Autodesk Inventor part; units mm, degrees
ref_plane "YZ Plane" through (0, 0, 0) normal (1, 0, 0) x (0, 1, 0)
ref_plane "XZ Plane" through (0, 0, 0) normal (0, 1, 0) x (-1, 0, 0)
ref_plane "XY Plane" through (0, 0, 0) normal (0, 0, 1) x (1, 0, 0)
sketch "Sketch1" plane through (0, 0, 0) normal (0, 0, 1) x (1, 0, 0)
  line L0 (-115, 162.5) -> (115, 162.5)
  line L1 (115, 162.5) -> (115, -162.5)
  line L2 (115, -162.5) -> (-115, -162.5)
  line L3 (-115, -162.5) -> (-115, 162.5)
  point P0 (0, 0)
  point P1 (0, 162.5)
  point P2 (-115, 0)
  dimension "d0" = 230
  dimension "d1" = 325
extrude "Extrusion1" add sketch "Sketch1" along normal blind 8
sketch "Sketch2" plane through (0, 0, 8) normal (0, 0, 1) x (1, 0, 0)
  line L0 (-110, -157.5) -> (110, -157.5) construction
  line L1 (110, -157.5) -> (110, 157.5) construction
  line L2 (110, 157.5) -> (-110, 157.5) construction
  line L3 (-110, 157.5) -> (-110, -157.5) construction
  line L4 (-115, 162.5) -> (-115, -162.5) construction
  line L5 (115, 162.5) -> (-115, 162.5) construction
  point P0 (0, 0)
  point P1 (-110, 0)
  point P2 (-115, 0)
  point P3 (-115, 0)
  point P4 (0, 157.5)
  point P5 (0, 162.5)
  dimension "d4" = 5
  dimension "d5" = 5
hole "Hole1" at (-110, -157.5, 8) at (-110, 157.5, 8) at (110, 157.5, 8) at (110, -157.5, 8) direction (0, 0, -1) diameter 3.5 end through all
sketch "Sketch3" plane through (0, 0, 8) normal (0, 0, 1) x (1, 0, 0)
  line L0 (65, -162.5) -> (-65, -162.5)
  line L1 (-65, -162.5) -> (-65, -25)
  line L2 (-65, -25) -> (65, -25)
  line L3 (65, -25) -> (65, -162.5)
  line L4 (-115, -162.5) -> (115, -162.5)
  line L5 (115, -162.5) -> (115, 162.5)
  line L6 (-115, 162.5) -> (-115, -162.5)
  line L7 (65, 25) -> (-65, 25)
  line L8 (-65, 25) -> (-65, 162.5)
  line L9 (-65, 162.5) -> (65, 162.5)
  line L10 (65, 162.5) -> (65, 25)
  line L11 (115, 162.5) -> (-115, 162.5)
  point P0 (0, 0)
  dimension "d13" = 50
  dimension "d14" = 50
  dimension "d15" = 25
  dimension "d16" = 25
extrude "Extrusion2" cut sketch "Sketch3" against normal blind 10 contours L0 L1 L2 L3 | L10 L7 L8 L9
sketch "Sketch4" plane through (0, 0, 8) normal (0, 0, 1) x (1, 0, 0)
  line L0 (-10, -15) -> (10, -15)
  line L1 (10, -15) -> (10, -5)
  line L2 (10, -5) -> (-10, -5)
  line L3 (-10, -5) -> (-10, -15)
  line L4 (-10, 5) -> (10, 5)
  line L5 (10, 5) -> (10, 15)
  line L6 (10, 15) -> (-10, 15)
  line L7 (-10, 15) -> (-10, 5)
  line L8 (-65, -25) -> (65, -25)
  line L9 (65, 25) -> (-65, 25)
  point P0 (0, 0)
  point P1 (0, -5)
  point P2 (0, 5)
  dimension "d19" = 10
  dimension "d20" = 10
  dimension "d21" = 10
  dimension "d22" = 20
extrude "Extrusion3" cut sketch "Sketch4" against normal through all
properties part number "0005-10-014 Suport Bed"
The model under review builds one solid part; all positions refer to its coordinate system, in mm. A direction names the side the tool comes from. Coordinates: 2 decimals unless noted, no trailing zeros. Order: outer loops, then holes, each group sorted by start corner. A loop starts at its lowest first (then second) coordinate and runs counter-clockwise, first axis right, second up. Notation, with made-up numbers: (69.25, 36) -> (107.25, 36) arc R11 ccw to (107.25, 48) -> close; hole circle Ø8 at (53, 63.5). An arc over 180 degrees is marked (long way). Answer in a Markdown table with one row per item.
(1) Consider section C-C (z = 5.75). Write out the cut boundary in (x, y), plus the area to 3 significant figures.
Answers:
| item | result |
|---|---|
| outline | (-115, -162.5) -> (-65, -162.5) -> (-65, -25) -> (65, -25) -> (65, -162.5) -> (115, -162.5) -> (115, 162.5) -> (65, 162.5) -> (65, 25) -> (-65, 25) -> (-65, 162.5) -> (-115, 162.5) -> close; hole circle Ø3.5 at (-110, -157.5); hole circle Ø3.5 at (-110, 157.5); hole (-10, -15) -> (10, -15) -> (10, -5) -> (-10, -5) -> close; hole (-10, 5) -> (10, 5) -> (10, 15) -> (-10, 15) -> close; hole circle Ø3.5 at (110, -157.5); hole circle Ø3.5 at (110, 157.5) |
| area | 38,600 mm² |
(2) Consider section A-A (y = -72.5). Write out the cut boundary in (x, z), plus the area to 3 significant figures.
Answers:
| item | result |
|---|---|
| outline | (-115, 0) -> (-65, 0) -> (-65, 8) -> (-115, 8) -> close; (65, 0) -> (115, 0) -> (115, 8) -> (65, 8) -> close |
| area | 800 mm² |
(3) Consider section B-B (x = 5). Write out the cut boundary in (y, z).
Answers:
| item | result |
|---|---|
| outline | (-25, 0) -> (-15, 0) -> (-15, 8) -> (-25, 8) -> close; (-5, 0) -> (5, 0) -> (5, 8) -> (-5, 8) -> close; (15, 0) -> (25, 0) -> (25, 8) -> (15, 8) -> close |
(4) Wall thickness on line 1 along Y through (x, z) = (-110, 4); line 2 along Y through (x, z) = (-1.5, 2.75); line 3 along X through (y, z) = (157.5, 5.25): over which ranges is each line inside the solid? List them lowest first.
Answers:
| item | result |
|---|---|
| line 1 | -162.5 to -159.25, -155.75 to 155.75, 159.25 to 162.5 |
| line 2 | -25 to -15, -5 to 5, 15 to 25 |
| line 3 | -115 to -111.75, -108.25 to -65, 65 to 108.25, 111.75 to 115 |
(5) Machinability: for faces 5 (the flat face through (0, -5, 4)), 6 (the flat face through (65, -93, 4)), 7 (the flat face through (90, 162.5, 4)), 8 (the flat face through (1, 25, 4)), 9 (the flat face through (90, -162.5, 4)), which of the approach directions +Z, -Z, +X, -X, +Y, -Y give a long, thin tool a straight path to every point of the face, cutting with its end or side? Answer none if there is none.
Answers:
| item | result |
|---|---|
| face 5 | +Z, -Z |
| face 6 | +Z, -Z, -Y |
| face 7 | +Z, -Z, +X, -X, +Y |
| face 8 | +Z, -Z, +Y |
| face 9 | +Z, -Z, +X, -X, -Y |
(6) The part is to be moulded in two halves that separate along X. For faces 1 (the flat face through (-1, -25, 4)), 2 (the flat face through (-2, 2, 0)), 3 (the flat face through (-115, -2, 4)), 4 (the flat face through (115, 2, 4)), say which applies: +X half, -X half, draft (parallel to the pull), parting line (faces both ways), or undercut.
Answers:
| item | result |
|---|---|
| face 1 | undercut |
| face 2 | draft |
| face 3 | -X half |
| face 4 | +X half |
(7) Insertion check: pin 1 (5 mm diameter, centred on x = -75.5, y = -55.5, fed in from -Z); pin 2 (3 mm diameter, centred on x = -110, y = 157.5, fed in from -Z) (3 decimals); pin 3 (4 mm diameter, centred on x = 3.5, z = 5, fed in from +Y); pin 4 (3 mm diameter, centred on x = -44.5, z = 5.5, fed in from -Y). Each pin has a flat end and moves straight along its axis. Give the tip position at first contact, or say it passes through.
Answers:
| item | result |
|---|---|
| pin 1 | z = 0 |
| pin 2 | through |
| pin 3 | y = 25 |
| pin 4 | y = -25 |
